from build123d import *

# Parameters (mm, degrees)
SKETCH3_W                     = 43.5
SKETCH3_H                     = 22
BOSS_EXTRUDE3_DEPTH           = 0.6
EDGE_FLANGE1_STRIP_W          = 3.6
EDGE_FLANGE1_STRIP_H          = 0.6
EDGE_FLANGE1_STRIP_CUT_DEPTH  = 3.155767649
EDGE_FLANGE1_RELIEF_W         = 3.9
EDGE_FLANGE1_RELIEF_H         = 0.3
EDGE_FLANGE1_RELIEF_CUT_DEPTH = 0.6
EDGE_FLANGE1_DEPTH            = 3.155767649


# Sheet-metal steps are written as plain solids
with BuildPart() as part:
    # Sketch3 → Boss-Extrude3 (new body)
    with BuildSketch(Plane.XY):
        with Locations((21.75, 11)):
            Rectangle(SKETCH3_W, SKETCH3_H)
    extrude(amount=BOSS_EXTRUDE3_DEPTH)

    # Edge-Flange1 strip (across the edge) → Edge-Flange1 strip cut (cut)
    with BuildSketch(Plane(origin=(0, 11.866760766, 0.6), x_dir=(1, 0, 0), z_dir=(0, -1, 0))):
        with Locations((-0.6, -0.3)):
            Rectangle(EDGE_FLANGE1_STRIP_W, EDGE_FLANGE1_STRIP_H)
    extrude(amount=EDGE_FLANGE1_STRIP_CUT_DEPTH, mode=Mode.SUBTRACT)

    # Edge-Flange1 relief (on the sheet) → Edge-Flange1 relief cut (cut)
    with BuildSketch(Plane(origin=(1.2, 11.866760766, 0.6), x_dir=(1, 0, 0), z_dir=(0, 0, 1))):
        with Locations((-1.65, 0.15)):
            Rectangle(EDGE_FLANGE1_RELIEF_W, EDGE_FLANGE1_RELIEF_H)
        with Locations((-1.65, -3.305767649)):
            Rectangle(EDGE_FLANGE1_RELIEF_W, EDGE_FLANGE1_RELIEF_H)
    extrude(amount=-EDGE_FLANGE1_RELIEF_CUT_DEPTH, mode=Mode.SUBTRACT)

    # Edge-Flange1 section (across the edge) → Edge-Flange1 (add)
    with BuildSketch(Plane(origin=(0, 11.866760766, 0.6), x_dir=(1, 0, 0), z_dir=(0, -1, 0))):
        with BuildLine():
            Line((0, 0.6), (0, 1.4))
            Line((0, 1.4), (0.6, 1.4))
            Line((0.6, 1.4), (0.6, 0.6))
            ThreePointArc((0.6, 0.6), (0.775735931, 0.175735931), (1.2, 0))
            Line((1.2, 0), (1.2, -0.6))
            ThreePointArc((1.2, -0.6), (0.351471863, -0.248528137), (0, 0.6))
        make_face()
    extrude(amount=EDGE_FLANGE1_DEPTH)


solid = part.part
Input: part model. Units: mm. Frame: model coordinates. A direction names the side the tool comes from. Coordinates: 2 decimals unless noted, no trailing zeros. Order: outer loops, then holes, each group sorted by start corner. A loop starts at its lowest first (then second) coordinate and runs counter-clockwise, first axis right, second up. Notation, with made-up numbers: M 14,41 L 50,41 A32 cw 50,79 Z; hole C -37.75,0 d7. An arc over 180 degrees is marked long. Answer in a Markdown table with one row per item.
(1) Section query B-B, the plane x = 18. Output: boundary loops of the cut face in (y, z), plus the area to 3 significant figures.
Numbers:
| item | result |
|---|---|
| outline | M 0,0 L 22,0 L 22,0.6 L 0,0.6 Z |
| area | 13.2 mm^2 |
(2) Draft query along Y for faces 1 (the flat face through (0.4, 11.867, 1)), 2 (the cylindrical face through (0.361, 10.311, 0.342)), 3 (the flat face through (21, 11, 0.6)). Return one class per face: pulls with the +Y half, pulls with the -Y half, needs draft (parallel to the pull), parting line crosses it, or undercut.
Numbers:
| item | result |
|---|---|
| face 1 | undercut |
| face 2 | undercut |
| face 3 | needs draft |
(3) Material intervals for line 1 (X direction, y = 10.25, z = 1.8), sorted ascending. Write a range as [from, to].
Numbers:
| item | result |
|---|---|
| line 1 | x = [0, 0.6] |
(4) Section query A-A, the plane z = 1.5. Output: boundary loops of the cut face in (x, y).
Numbers:
| item | result |
|---|---|
| outline | M 0,8.71 L 0.6,8.71 L 0.6,11.87 L 0,11.87 Z |
(5) Access query for faces 4 (the flat face through (0.4, 8.711, 1)), 5 (the flat face through (21, 11, 0)). Directions: +Z, -Z, +X, -X, +Y, -Y. A direction counts if a zero-diameter tool reaches every point of the face in a straight line with its end or side. Return the directions, or none.
Numbers:
| item | result |
|---|---|
| face 4 | +Z, -Z, -X |
| face 5 | -Z, +X, -X, +Y, -Y |
(6) Contact query for a flat-ended pin moving along its axis: pin 1 Ø11 at (x, y) = (22.5, 16.5) entering from +Z. Output: stop coordinate, or through.
Numbers:
| item | result |
|---|---|
| pin 1 | stops at z = 0.6 |
